from build123d import *

# Parameters (mm, degrees)
EXTRUDE_1_DEPTH     = 60
SKETCH_3_R          = 12
EXTRUDE_2_DEPTH     = 46
SKETCH_6_R          = 10
CUT_EXTRUDE_1_DEPTH = 69.381284144
SKETCH_7_R          = 8
CUT_EXTRUDE_2_DEPTH = 79.204859286
SKETCH_8_R          = 10
CUT_EXTRUDE_3_DEPTH = 77.655071751


with BuildPart() as part:
    # 草图1 → 凸台-拉伸1 (new body)
    with BuildSketch(Plane(origin=(0, 0, 0), x_dir=(0, 0, -1), z_dir=(1, 0, 0))):
        with BuildLine():
            Line((-20, 0), (-20, -20))
            Line((-20, -20), (20, -20))
            Line((20, -20), (20, 0))
            ThreePointArc((20, 0), (0, 20), (-20, 0))
        make_face()
    extrude(amount=EXTRUDE_1_DEPTH)

    # 草图3 → 凸台-拉伸2 (add)
    with BuildSketch(Plane(origin=(0, -20, 0), x_dir=(-1, 0, 0), z_dir=(0, -1, 0))):
        with Locations(Location((-40, 0, 0), (0, 0, 90))):
            Circle(SKETCH_3_R)
    extrude(amount=-EXTRUDE_2_DEPTH)

    # 草图6 → 切除-拉伸1 (cut, through all)
    with BuildSketch(Plane.ZY):
        Circle(SKETCH_6_R)
    extrude(amount=-CUT_EXTRUDE_1_DEPTH, mode=Mode.SUBTRACT)

    # 草图7 → 切除-拉伸2 (cut, through all)
    with BuildSketch(Plane(origin=(0, 26, 0), x_dir=(1, 0, 0), z_dir=(0, 1, 0))):
        with Locations(Location((40, 0, 0), (0, 0, 270))):
            Circle(SKETCH_7_R)
    extrude(amount=-CUT_EXTRUDE_2_DEPTH, mode=Mode.SUBTRACT)

    # 草图8 → 切除-拉伸3 (cut, through all)
    with BuildSketch(Plane.XY.offset(20)):
        with Locations((20, 0)):
            Circle(SKETCH_8_R)
    extrude(amount=-CUT_EXTRUDE_3_DEPTH, mode=Mode.SUBTRACT)


solid = part.part
Build history of the part. All positions in model axes, mm. A direction names the side the tool comes from. Coordinates: 2 decimals unless noted, no trailing zeros. Order: outer loops, then holes, each group sorted by start corner. A loop starts at its lowest first (then second) coordinate and runs counter-clockwise, first axis right, second up. Notation, with made-up numbers: M 27,82 L 83,82 A36 ccw 83,117 Z; hole C 3.5,0.25 d10. An arc over 180 degrees is marked long. One line per question, with ' | ' between items. Start each with the question number.
Q1. Saw through at C-C (x = 6). List the corners of the cut face in (y, z).
Q2. Two-plate mould, pull along X, no slides. Class faces 3 (the face through (0, -13, 0)), 4 (the face through (30, -10, -20)), 5 (the face through (24.614, -8.872, 12.362)): +X half, -X half, draft (parallel to the pull), parting line (faces both ways), or undercut.
Q3. Flat gauge pins, fed straight in: pin 1 Ø4 at (y, z) = (13.5, -6) entering from -X; pin 2 Ø18 at (x, y) = (20, 0) entering from +Z; pin 3 Ø1.5 at (x, y) = (48, 7.5) entering from -Z; pin 4 Ø4 at (x, y) = (45, 7.5) entering from +Z. Where does each tip first touch, or does it go through?
Q4. Saw through at A-A (x = 37). List the corners of the cut face in (y, z).
Q5. 3-axis set-ups, long thin cutter, end or side, ignore diameter. For faces 1 (the face through (32.698, 22.041, 9.523)), 2 (the face through (32, 26, -2)): which of +Z, -Z, +X, -X, +Y, -Y reach the whole face in a straight line?
Q6. Saw through at B-B (z = -4.5). List the corners of the cut face in (x, y), then the cut area to 3 significant figures.
Q7. Saw through at D-D (z = 13). List the corners of the cut face in (x, y).
Q8. Probe L1, parallel to X at y = 0, z = 15.5; L2, parallel to Z at x = 33.5, y = 9; L3, parallel to Y at x = 20, z = -8. List the from-to ranges inside material, lowest first. Write a range as from..to.
Check values:
1) outline: M -20,-20 L 0,-20 A20 ccw 0,20 L -20,20 Z; hole C 0,0 d20
2) face 3: -X half | face 4: draft | face 5: undercut
3) pin 1: stops at x = 0 | pin 2: passes through | pin 3: stops at z = -18.83 | pin 4: stops at z = 19.23
4) outline: M -20,-20 L 0,-20 A20 ccw 16.28,-11.62 L 26,-11.62 L 26,-7.42 L 6.71,-7.42 A10 cw -6.71,-7.42 L -20,-7.42 Z; M -20,7.42 L -6.71,7.42 A10 cw 6.71,7.42 L 26,7.42 L 26,11.62 L 16.28,11.62 A20 ccw 0,20 L -20,20 Z
5) face 1: +Y | face 2: +Z, -Z, +X, -X, +Y
6) outline: M 0,-20 L 33.39,-20 L 33.39,-8.93 L 24.5,-8.93 A10 cw 15.5,-8.93 L 0,-8.93 Z; M 0,8.93 L 15.5,8.93 A10 cw 24.5,8.93 L 33.39,8.93 L 33.39,26 L 28.88,26 L 28.88,19.49 L 0,19.49 Z; M 46.61,-20 L 60,-20 L 60,-8.93 L 46.61,-8.93 Z; M 46.61,8.93 L 60,8.93 L 60,19.49 L 51.12,19.49 L 51.12,26 L 46.61,26 Z | area: 1,060 mm2
7) outline: M 0,-20 L 60,-20 L 60,15.2 L 0,15.2 Z; hole C 20,0 d20
8) L1: x = 0..10, 30..60 | L2: z = -17.86..-4.66, 4.66..17.86 | L3: y = -20..-10, 10..18.33
